Build history of the part. All positions in model axes, mm. A direction names the side the tool comes from. Round coordinates to 2 decimals unless told otherwise and drop trailing zeros. Write each loop counter-clockwise with the first axis right and the second up, starting at its lowest first coordinate (ties: lowest second). Pieces come first, ordered by that corner, then holes. Notation, with made-up numbers: M -30,4.5 L -10,4.5 A32 ccw -10,39.5 Z; hole C -26,84 d3. An arc over 180 degrees is marked long. Use a Markdown table: item, result.
from build123d import *

# Parameters (mm, degrees)
BOSS_EXTRUDE2_DEPTH      = 29
BOSS_EXTRUDE2_DEPTH_BACK = 2
SKETCH1_R                = 3.5
BOSS_EXTRUDE3_DEPTH      = 4.5
BOSS_EXTRUDE3_DEPTH_BACK = 4.5
SKETCH2_R                = 12
SKETCH2_R_2              = 7


# Read off the part's stored shape, not the designer's step: Cut-Revolve-Thin4
with BuildPart() as part:
    # Sketch1 → Boss-Extrude2 (new, two sides: drawn at the far end of the back side and taken through both)
    with BuildSketch(Plane.YZ.offset(-BOSS_EXTRUDE2_DEPTH_BACK)):
        with Locations(Location((0, 0, 0), (0, 0, 270))):
            Circle(SKETCH1_R)
    extrude(amount=BOSS_EXTRUDE2_DEPTH + BOSS_EXTRUDE2_DEPTH_BACK)

    # Sketch2 → Boss-Extrude3 (add, two sides: drawn at the far end of the back side and taken through both)
    with BuildSketch(Plane(origin=(0, 0, 0), x_dir=(-1, 0, 0), z_dir=(0, 1, 0)).offset(-BOSS_EXTRUDE3_DEPTH_BACK)):
        with Locations(Location((12, 0, 0), (0, 0, 90))):
            Circle(SKETCH2_R)
        with Locations(Location((12, 0, 0), (0, 0, 90))):
            Circle(SKETCH2_R_2, mode=Mode.SUBTRACT)
    extrude(amount=BOSS_EXTRUDE3_DEPTH + BOSS_EXTRUDE3_DEPTH_BACK)

    # Cut-Revolve-Thin4 outline → Cut-Revolve-Thin4 (revolve, cut)
    with BuildSketch(Plane(origin=(-12, 0, 0), x_dir=(1, 0, 0), z_dir=(0, 0, 1))):
        with BuildLine():
            Line((6.999999996, 4.459820631), (6.999999996, -4.459820631))
            ThreePointArc((6.999999996, -4.459820631), (8.3, 0), (6.999999996, 4.459820631))
        make_face()
    revolve(axis=Axis((-12, 0, 0), (0, 1, 0)), mode=Mode.SUBTRACT)


solid = part.part
Q1. Drop flat-ended pins along their axis: P1, Ø5, axis at x = 17, z = 3, coming from the +Y side; P2, Ø1.5, axis at x = 5.5, y = 0.5, coming from the +Z side. Give the stop position or say it passes through.
Response values:
| item | result |
|---|---|
| P1 | stops at y = 3.46 |
| P2 | stops at z = 3.5 |
Q2. Cut at C-C on y = 0. Give the cut face in (x, z).
Response values:
| item | result |
|---|---|
| outline | M -0.52,-3.5 L 29,-3.5 L 29,3.5 L -0.52,3.5 A12 ccw long Z; hole C -12,0 d16.6 |
Q3. Cut at D-D on z = -7.5. Give the cut face in (x, y), and give its area (3 significant figures).
Response values:
| item | result |
|---|---|
| outline | M -21.37,-4.5 L -2.63,-4.5 L -2.63,4.5 L -21.37,4.5 Z; hole C -12,0 d7.11 |
| area | 129 mm2 |
Q4. Cut at A-A on z = 0. Give the cut face in (x, y).
Response values:
| item | result |
|---|---|
| outline | M -24,-4.5 L -19,-4.5 L -19,-4.46 A8.3 cw -19,4.46 L -19,4.5 L -24,4.5 Z; M -5,-4.5 L 0,-4.5 L 0,-3.5 L 29,-3.5 L 29,3.5 L 0,3.5 L 0,4.5 L -5,4.5 L -5,4.46 A8.3 cw -5,-4.46 Z |
Q5. Drill centre lines: L1, parallel to X at y = -4.45, z = 0; L2, parallel to Z at x = -19, y = -3; L3, parallel to Z at x = -10, y = 2.75. Where is each one in solid material? Low to high.
Response values:
| item | result |
|---|---|
| L1 | x = -24 to -19.01, -4.99 to 0 |
| L2 | z = -9.75 to -3.3, 3.3 to 9.75 |
| L3 | z = -11.83 to -7.57, 7.57 to 11.83 |
Q6. Cut at B-B on x = -12. Give the cut face in (y, z).
Response values:
| item | result |
|---|---|
| outline | M -4.5,-12 L 4.5,-12 L 4.5,-7 L 4.46,-7 A8.3 cw -4.46,-7 L -4.5,-7 Z; M -4.5,7 L -4.46,7 A8.3 cw 4.46,7 L 4.5,7 L 4.5,12 L -4.5,12 Z |
Q7. Which spindle directions (+Z, -Z, +X, -X, +Y, -Y) get a long thin tool onto all of the face, cutting with end or side? Do faces 1 (the cylindrical face through (14.017, -3.417, 0.759)), 2 (the flat face through (-17.2, 4.5, 5.2)). Say none if no direction does.
Response values:
| item | result |
|---|---|
| face 1 | +X |
| face 2 | +Z, -Z, +X, -X, +Y |
